Geometry: final body of the model. Coordinates: model frame, mm. Face numbers are marked on the shaded views. Give positions to 0.01 mm unless a question says otherwise; leave off trailing zeros. Order: outer loops, then holes, each group sorted by start corner. A loop starts at its lowest first (then second) coordinate and runs counter-clockwise, first axis right, second up. Notation, with made-up numbers: (10, 84) - (50, 84) arc R16 ccw to (50, 108) - close; hole circle Ø1 at (73.5, 52). An arc over 180 degrees is marked (long way). One line per item, written item: value.
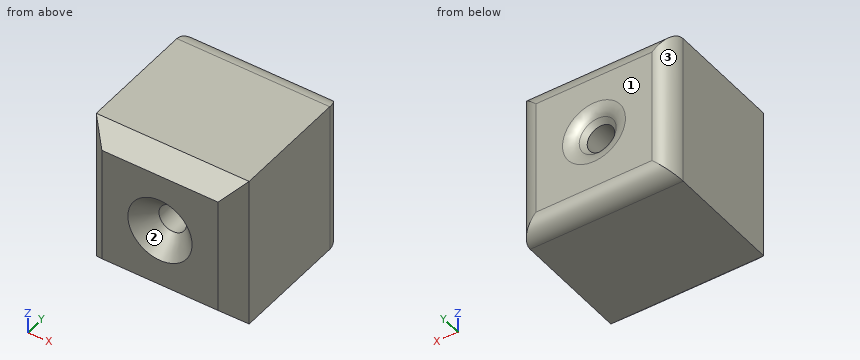
```python
from build123d import *

# Parameters (mm, degrees)
SKETCH_1_W      = 25
SKETCH_1_H      = 25
EXTRUDE_1_DEPTH = 25
FILLET_1_R      = 3
CHAMFER_1_SIZE  = 3


with BuildPart() as part:
    # 草图1 → 凸台-拉伸1 (new body)
    with BuildSketch(Plane.XY):
        with Locations((12.5, 12.5)):
            Rectangle(SKETCH_1_W, SKETCH_1_H)
    extrude(amount=EXTRUDE_1_DEPTH)

    # 草图3 → 切除-旋转1 (revolve, cut)
    with BuildSketch(Plane.XY.offset(12.5), mode=Mode.PRIVATE) as cut_revolve_1_sk:
        Polygon((10.25, 23.35), (10.25, 0), (12.5, 0), (12.5, 25), (8.6, 25), align=None)
    revolve(cut_revolve_1_sk.sketch.rotate(Axis((12.5, 25, 12.5), (0, -1, 0)), 270), axis=Axis((12.5, 25, 12.5), (0, -1, 0)), mode=Mode.SUBTRACT)

    # 圆角1
    fillet_1_edges = [part.edges().sort_by_distance(p)[0] for p in [
        (12.5, 25, 25),
        (12.5, 25, 8.6),
        (12.5, 25, 0),
        (0, 25, 12.5),
        (25, 25, 12.5),
    ]]
    fillet(fillet_1_edges, radius=FILLET_1_R)

    # 倒角1
    chamfer_1_edges = [part.edges().sort_by_distance(p)[0] for p in [
        (12.5, 0, 10.25),
        (12.5, 0, 0),
        (25, 0, 12.5),
        (0, 0, 12.5),
        (12.5, 0, 25),
    ]]
    chamfer(chamfer_1_edges, length=CHAMFER_1_SIZE)


solid = part.part
```
1) Mould query, pull axis X, two halves, no side actions, for the marked faces 1, 2 and 3. Classes: released by +X, released by -X, zero draft, split by the parting line, or undercut.
Answers below:
face 1: zero draft
face 2: undercut
face 3: released by -X
2) Section C-C, the plane x = 12.5. Return loops of the section in (y, z), then the cut area to 3 significant figures.
Answers below:
outline: (0, 3) - (3, 0) - (22, 0) arc R3 ccw to (25, 3) - (25, 7.36) arc R3 ccw to (24.12, 9.48) - (23.35, 10.25) - (3, 10.25) - (0, 7.25) - close; (0, 17.75) - (3, 14.75) - (23.35, 14.75) - (24.12, 15.52) arc R3 ccw to (25, 17.64) - (25, 22) arc R3 ccw to (22, 25) - (3, 25) - (0, 22) - close
area: 488 mm^2
3) Section A-A, the plane z = 12.5. Return loops of the section in (x, y), then the cut area to 3 significant figures.
Answers below:
outline: (0, 3) - (3, 0) - (7.25, 0) - (10.25, 3) - (10.25, 23.35) - (9.48, 24.12) arc R3 ccw to (7.36, 25) - (3, 25) arc R3 ccw to (0, 22) - close; (14.75, 3) - (17.75, 0) - (22, 0) - (25, 3) - (25, 22) arc R3 ccw to (22, 25) - (17.64, 25) arc R3 ccw to (15.52, 24.12) - (14.75, 23.35) - close
area: 488 mm^2
4) Section B-B, the plane y = 11.5. Return loops of the section in (x, z).
Answers below:
outline: (0, 0) - (25, 0) - (25, 25) - (0, 25) - close; hole circle Ø4.5 at (12.5, 12.5)
5) Material intervals for line 1 along X through (y, z) = (11.5, 12.5); line 2 along Z through (x, y) = (11.5, 7.5); line 3 along Z through (x, y) = (10.5, 2), sorted ascending.
Answers below:
line 1: 0 to 10.25, 14.75 to 25
line 2: 0 to 10.48, 14.52 to 25
line 3: 1 to 9.94, 15.06 to 24
6) First-contact query: pin 1 (5 mm diameter, centred on x = 12.5, z = 12.5, fed in from +Y); pin 2 (5 mm diameter, centred on x = 13.5, z = 15, fed in from +Y). Flat tips, straight axial feed; report the tip coordinate or a pass-through.
Answers below:
pin 1: y = 23.6
pin 2: y = 25
7) Section D-D, the plane z = 3.5. Return loops of the section in (x, y).
Answers below:
outline: (0, 3) - (3, 0) - (22, 0) - (25, 3) - (25, 22) arc R3 ccw to (22, 25) - (3, 25) arc R3 ccw to (0, 22) - close
